from build123d import *

# Parameters (mm, degrees)
CHANFREIN1_SIZE       = 0.4
EXTRUSION1_DEPTH      = 29.380374565
EXTRUSION1_DEPTH_BACK = 29.380374565
ESQUISSE2_W           = 6.7
ESQUISSE2_H           = 0.2


with BuildPart() as part:
    # Esquisse1 → Révolution1 (revolve)
    with BuildSketch(Plane.XY, mode=Mode.PRIVATE) as r_volution1_sk:
        Polygon((-22.272213686, 0), (-22.272213686, 8), (8.327786314, 8), (8.327786314, 7.25), (10.327786314, 7.25), (10.327786314, 8), (11.827786314, 8), (11.827786314, 3.5), (13.327786314, 3.5), (13.327786314, 3.111665859), (14.127786314, 3.111665859), (14.127786314, 1.5), (26.027786314, 1.5), (26.027786314, 0), align=None)
    revolve(r_volution1_sk.sketch.rotate(Axis((-64.659997946, 0, 0), (1, 0, 0)), 90), axis=Axis((-64.659997946, 0, 0), (1, 0, 0)))

    # Chanfrein1
    chanfrein1_edges = [part.edges().sort_by_distance(p)[0] for p in [
        (8.327786314, 0, -8),
    ]]
    chamfer(chanfrein1_edges, length=CHANFREIN1_SIZE)

    # Esquisse2 → Extrusion1 (cut, two sides: drawn at the far end of the back side and taken through both)
    with BuildSketch(Plane.XY.offset(-EXTRUSION1_DEPTH_BACK)):
        with Locations((18.377786314, 1.4)):
            Rectangle(ESQUISSE2_W, ESQUISSE2_H)
    extrude(amount=EXTRUSION1_DEPTH + EXTRUSION1_DEPTH_BACK, mode=Mode.SUBTRACT)


solid = part.part
Check sheet for the modelled part. Datum: model origin and axes. Units: mm. A direction names the side the tool comes from. Give positions to 0.01 mm unless a question says otherwise; leave off trailing zeros. Loops run counter-clockwise (first coordinate to the right, second up) from the corner with the lowest first, then second, coordinate; pieces in that order, holes last. Notation, with made-up numbers: M 81.5,23 L 88.5,23 A33 cw 88.5,55 Z; hole C 52.5,2.5 d7. An arc over 180 degrees is marked long. Return JSON: item names as keys, results as strings. Group by question number.
1. Thickness scan on L1, parallel to X at y = -2.5, z = -7; L2, parallel to X at y = 5, z = 1.25; L3, parallel to X at y = 2.5, z = -0.5. Record the ranges inside material, lowest first.
2. Cross-section at A-A on y = 0. Record the boundary of the cut face in (x, z), plus the area to 3 significant figures.
3. Tool access check on faces 1 (the cylindrical face through (13.73, 3.04, -0.67)), 2 (the flat face through (26.028, 0, 0)), 3 (the flat face through (18, 1.3, 0)). Record the directions out of +Z, -Z, +X, -X, +Y, -Y that give a thin tool (end or side, any length) a straight path to the whole face; none if there is none.
4. Cross-section at C-C on x = 4.5. Record the boundary of the cut face in (y, z), plus the area to 3 significant figures.
5. Go/stop test with flat-tipped pins: pin 1 (1.5 mm diameter, centred on y = 5.5, z = -2.5, fed in from +X); pin 2 (8 mm diameter, centred on x = -17.5, y = 6.5, fed in from +Z); pin 3 (3 mm diameter, centred on x = -15.5, y = 2, fed in from -Z). Record where each tip stops, or that it passes through.
6. Mould release check, pull along X, two halves, no side actions. Record for faces 4 (the cylindrical face through (9.34, 6.43, 3.35)), 5 (the cylindrical face through (11.09, 7.81, -1.73)), 6 (the flat face through (-22.272, 0, 0)): released by +X, released by -X, zero draft, split by the parting line, or undercut.
7. Cross-section at D-D on x = 17.5. Record the boundary of the cut face in (y, z).
Return value:
{
 "1": {"L1": "-22.27 to 8.33, 10.33 to 11.83", "L2": "-22.27 to 11.83", "L3": "-22.27 to 14.13"},
 "2": {"outline": "M -22.27,-8 L 7.93,-8 L 8.33,-7.6 L 8.33,-7.25 L 10.33,-7.25 L 10.33,-8 L 11.83,-8 L 11.83,-3.5 L 13.33,-3.5 L 13.33,-3.11 L 14.13,-3.11 L 14.13,-1.5 L 26.03,-1.5 L 26.03,1.5 L 14.13,1.5 L 14.13,3.11 L 13.33,3.11 L 13.33,3.5 L 11.83,3.5 L 11.83,8 L 10.33,8 L 10.33,7.25 L 8.33,7.25 L 8.33,7.6 L 7.93,8 L -22.27,8 Z", "area": "594 mm^2"},
 "3": {"face 1": "+X", "face 2": "+Z, -Z, +X, +Y, -Y", "face 3": "+Z, -Z, +Y"},
 "4": {"outline": "C 0,0 d16", "area": "201 mm^2"},
 "5": {"pin 1": "x = 11.83", "pin 2": "z = 7.6", "pin 3": "z = -7.98"},
 "6": {"face 4": "undercut", "face 5": "zero draft", "face 6": "released by -X"},
 "7": {"outline": "M 1.3,-0.75 L 1.3,0.75 A1.5 ccw long Z"}
}
